Source: CAD feature listing. Evaluate the final solid. Frame: model axes, mm. A direction names the side the tool comes from. Give positions to 0.01 mm unless a question says otherwise; leave off trailing zeros. Order: outer loops, then holes, each group sorted by start corner. A loop starts at its lowest first (then second) coordinate and runs counter-clockwise, first axis right, second up. Notation, with made-up numbers: (14.5, 40.25) - (47.5, 40.25) arc R10 ccw to (47.5, 52.25) - close; hole circle Ø11 at (42, -28.75). An arc over 180 degrees is marked (long way). Answer as CSV lines item,"result".
```python
from build123d import *

# Parameters (mm, degrees)
F1_DEPTH    = 19.05
F2_W        = 10.287
F2_H        = 5.9704589657
F2_W_2      = 10.7644796371
F3_DEPTH    = 3.048
F4_T1_DEPTH = 69.8499994576
F4_T3_DEPTH = 187.4519989152


# Not quite as in the source:
# - a fillet or chamfer that OpenCascade refuses, or shapes differently, is made with other operations: its cross-section is extruded or revolved along the edge and cut away or added


with BuildPart() as f1:
    # F0 (on Front) → F1 (new body)
    with BuildSketch(Plane.XZ):
        Polygon((-38.0874201655, -5.7323638652), (-38.0874201655, 19.6676361348), (-44.4374196231, 19.6676361348), (-44.4374196231, -12.0823633227), (104.9145792921, -12.0823633227), (104.9145792921, 19.6676361348), (98.5645798345, 19.6676361348), (98.5645798345, -5.7323638652), align=None)
    extrude(amount=F1_DEPTH)

    # F2 (on Front) → F3 (join)
    with BuildSketch(Plane.XZ):
        with Locations((-32.9439201655, -2.9852294829)):
            Rectangle(F2_W, F2_H)
        with Locations((93.29213202, -2.9852294829)):
            Rectangle(F2_W_2, F2_H)
    extrude(amount=F3_DEPTH)

    # F4: fillet of radius 7.62 on 3 edges, made by hand

    # F4_s2 → F4_t1 (cut)
    with BuildSketch(Plane.XY.offset(-31.1323633227)):
        with BuildLine():
            ThreePointArc((97.2945792921, 0), (102.6827329647, -2.2318463274), (104.9145792921, -7.62))
            Line((104.9145792921, -7.62), (104.9145792921, 0))
            Line((104.9145792921, 0), (97.2945792921, 0))
        make_face()
        with BuildLine():
            ThreePointArc((-36.8174196231, 0), (-42.2055732958, -2.2318463274), (-44.4374196231, -7.62))
            Line((-44.4374196231, -7.62), (-44.4374196231, 0))
            Line((-44.4374196231, 0), (-36.8174196231, 0))
        make_face()
    extrude(amount=F4_T1_DEPTH, mode=Mode.SUBTRACT)

    # F4_s4 → F4_t3 (cut)
    with BuildSketch(Plane.YZ.offset(-63.4874196231)):
        with BuildLine():
            ThreePointArc((0, -4.4623633227), (-2.2318463274, -9.8505169954), (-7.62, -12.0823633227))
            Line((-7.62, -12.0823633227), (0, -12.0823633227))
            Line((0, -12.0823633227), (0, -4.4623633227))
        make_face()
    extrude(amount=F4_T3_DEPTH, mode=Mode.SUBTRACT)


solid = f1.part
```
(1) Cut plane D-D (x = 71). Return loops of the section in (y, z), then the cut area to 3 significant figures.
Completed:
outline,"(-19.05, -12.08) - (-7.62, -12.08) arc R7.62 ccw to (-0.11, -5.73) - (-19.05, -5.73) - close"
area,"109 mm²"
(2) Access query for faces 1 (the flat face through (-27.8, -2, -3)), 2 (the flat face through (-38.087, -9, 7)), 3 (the flat face through (29, -13, -12.082)). Directions: +Z, -Z, +X, -X, +Y, -Y. A direction counts if a zero-diameter tool reaches every point of the face in a straight line with its end or side. Return the directions, or none.
Completed:
face 1,"+Z, +Y, -Y"
face 2,"+Z, -Y"
face 3,"-Z, +X, -X, +Y, -Y"
(3) Mould query, pull axis X, two halves, no side actions, for faces 4 (the flat face through (87.91, -2, -3)), 5 (the flat face through (31, -9, -5.732)), 6 (the cylindrical face through (-43.01, -3.18, 3.57)), 7 (the cylindrical face through (103.5, -3.2, 3.6)). Classes: released by +X, released by -X, zero draft, split by the parting line, or undercut.
Completed:
face 4,"undercut"
face 5,"undercut"
face 6,"released by -X"
face 7,"released by +X"
(4) Ray query, line 1 (X direction, y = -12.5, z = 1); line 2 (Z direction, x = 61, y = -15.75); line 3 (X direction, y = -1.25, z = 10.5). Return the intervals inside material, ascending. Write a range as from..to.
Completed:
line 1,"-44.44..-38.09, 98.56..104.91"
line 2,"-12.08..-5.73"
line 3,"-41..-38.09, 98.56..101.48"
(5) Cut plane B-B (y = -16). Return loops of the section in (x, z).
Completed:
outline,"(-44.44, -12.08) - (104.91, -12.08) - (104.91, 19.67) - (98.56, 19.67) - (98.56, -5.73) - (-38.09, -5.73) - (-38.09, 19.67) - (-44.44, 19.67) - close"
(6) Contact query for flat-ended pins moving along their axis: pin 1 (5 mm diameter, centred on x = 38.5, y = -15, fed in from +Z); pin 2 (1.5 mm diameter, centred on y = -1.5, z = -4, fed in from -X); pin 3 (3 mm diameter, centred on x = 93.5, z = -3, fed in from -Y). Output: stop coordinate, or through.
Completed:
pin 1,"z = -5.73"
pin 2,"x = -42.22"
pin 3,"y = -3.05"
(7) Cut plane A-A (z = 7). Return loops of the section in (x, y), then the cut area to 3 significant figures.
Completed:
outline,"(-44.44, -19.05) - (-38.09, -19.05) - (-38.09, -0.11) arc R7.62 ccw to (-44.44, -7.62) - close; (98.56, -19.05) - (104.91, -19.05) - (104.91, -7.62) arc R7.62 ccw to (98.56, -0.11) - close"
area,"217 mm²"
(8) Cut plane C-C (z = -2.5). Return loops of the section in (x, y).
Completed:
outline,"(-44.44, -19.05) - (-38.09, -19.05) - (-38.09, -3.05) - (-27.8, -3.05) - (-27.8, 0) - (-36.82, 0) arc R7.62 ccw to (-44.44, -7.62) - close; (87.91, -3.05) - (98.56, -3.05) - (98.56, -19.05) - (104.91, -19.05) - (104.91, -7.62) arc R7.62 ccw to (97.29, 0) - (87.91, 0) - close"
